```python
from build123d import *

# Parameters (mm, degrees)
CROQUIS1_W              = 60.5
CROQUIS1_H              = 54.5
SALIENTE_EXTRUIR1_DEPTH = 25
CROQUIS2_W              = 56.9
CROQUIS2_H              = 50.9
CORTAR_EXTRUIR1_DEPTH   = 15
CROQUIS3_R              = 2.1
CORTAR_EXTRUIR2_DEPTH   = 5
CORTAR_EXTRUIR3_DEPTH   = 5
CORTAR_EXTRUIR4_DEPTH   = 1.8
CORTAR_EXTRUIR6_START   = -1.8
CORTAR_EXTRUIR6_DEPTH   = 60.5
CROQUIS10_W             = 6
CROQUIS10_H             = 6
CROQUIS10_R             = 1.6
SALIENTE_EXTRUIR2_DEPTH = 3
CROQUIS11_W             = 58.5
CROQUIS11_H             = 52.5
CORTAR_EXTRUIR7_DEPTH   = 15


with BuildPart() as part:
    # Croquis1 → Saliente-Extruir1 (new body)
    with BuildSketch(Plane.XY):
        with Locations((-43.305557703, 3.094674556)):
            Rectangle(CROQUIS1_W, CROQUIS1_H)
    extrude(amount=SALIENTE_EXTRUIR1_DEPTH)

    # Croquis2 → Cortar-Extruir1 (cut)
    with BuildSketch(Plane.XY.offset(25)):
        with Locations((-43.305557703, 3.094674556)):
            Rectangle(CROQUIS2_W, CROQUIS2_H)
    extrude(amount=-CORTAR_EXTRUIR1_DEPTH, mode=Mode.SUBTRACT)

    # Croquis3 → Cortar-Extruir2 (cut)
    with BuildSketch(Plane.XY.offset(10)):
        with Locations((-68.955557703, 25.744674556)):
            Circle(CROQUIS3_R)
        with Locations((-55.855557703, -19.355325444)):
            Circle(CROQUIS3_R)
        with Locations((-30.755557703, -19.355325444)):
            Circle(CROQUIS3_R)
        with Locations((-17.655557703, 25.744674556)):
            Circle(CROQUIS3_R)
        Polygon((-71.755557703, 20.544674556), (-71.755557703, -22.355325444), (-59.855557703, -22.355325444), (-59.855557703, -14.355325444), (-51.855557703, -14.355325444), (-51.855557703, -22.355325444), (-34.755557703, -22.355325444), (-34.755557703, -14.355325444), (-26.755557703, -14.355325444), (-26.755557703, -22.355325444), (-14.855557703, -22.355325444), (-14.855557703, 20.544674556), (-22.855557703, 20.544674556), (-22.855557703, 28.544674556), (-63.755557703, 28.544674556), (-63.755557703, 20.544674556), align=None)
    extrude(amount=-CORTAR_EXTRUIR2_DEPTH, mode=Mode.SUBTRACT)

    # Croquis5 → Cortar-Extruir3 (cut)
    with BuildSketch(Plane(origin=(0, -22.355325444, 0), x_dir=(1, 0, 0), z_dir=(0, 1, 0))):
        with BuildLine():
            Line((-18.605557703, -18), (-18.605557703, -25))
            Line((-18.605557703, -25), (-26.105557703, -25))
            Line((-26.105557703, -25), (-26.105557703, -18))
            ThreePointArc((-26.105557703, -18), (-22.355557703, -14.25), (-18.605557703, -18))
        make_face()
        with BuildLine():
            Line((-39.605557703, -18), (-39.605557703, -25))
            Line((-39.605557703, -25), (-47.105557703, -25))
            Line((-47.105557703, -25), (-47.105557703, -18))
            ThreePointArc((-47.105557703, -18), (-43.355557703, -14.25), (-39.605557703, -18))
        make_face()
        with BuildLine():
            Line((-60.605557703, -18), (-60.605557703, -25))
            Line((-60.605557703, -25), (-68.105557703, -25))
            Line((-68.105557703, -25), (-68.105557703, -18))
            ThreePointArc((-68.105557703, -18), (-64.355557703, -14.25), (-60.605557703, -18))
        make_face()
    extrude(amount=-CORTAR_EXTRUIR3_DEPTH, mode=Mode.SUBTRACT)

    # Croquis6 → Cortar-Extruir4 (cut)
    with BuildSketch(Plane.XZ.offset(-28.544674556)):
        Polygon((-64.805557703, 17), (-21.805557703, 17), (-21.805557703, 10), (-22.855557703, 10), (-22.855557703, 5), (-30.855557703, 5), (-30.855557703, 10), (-64.805557703, 10), align=None)
    extrude(amount=-CORTAR_EXTRUIR4_DEPTH, mode=Mode.SUBTRACT)

    # Croquis9 → Cortar-Extruir6 (cut)
    with BuildSketch(Plane(origin=(-71.755557703, 0, 0), x_dir=(0, 0, -1), z_dir=(1, 0, 0)).offset(CORTAR_EXTRUIR6_START)):
        with BuildLine():
            Line((-10, 20.544674556), (-20, 20.544674556))
            ThreePointArc((-20, 20.544674556), (-22.5, 18.044674556), (-20, 15.544674556))
            Line((-20, 15.544674556), (-10, 15.544674556))
            ThreePointArc((-10, 15.544674556), (-7.5, 18.044674556), (-10, 20.544674556))
        make_face()
        with BuildLine():
            Line((-10, 10.544674556), (-20, 10.544674556))
            ThreePointArc((-20, 10.544674556), (-22.5, 8.044674556), (-20, 5.544674556))
            Line((-20, 5.544674556), (-10, 5.544674556))
            ThreePointArc((-10, 5.544674556), (-7.5, 8.044674556), (-10, 10.544674556))
        make_face()
        with BuildLine():
            Line((-10, 0.544674556), (-20, 0.544674556))
            ThreePointArc((-20, 0.544674556), (-22.5, -1.955325444), (-20, -4.455325444))
            Line((-20, -4.455325444), (-10, -4.455325444))
            ThreePointArc((-10, -4.455325444), (-7.5, -1.955325444), (-10, 0.544674556))
        make_face()
        with BuildLine():
            Line((-10, -9.455325444), (-20, -9.455325444))
            ThreePointArc((-20, -9.455325444), (-22.5, -11.955325444), (-20, -14.455325444))
            Line((-20, -14.455325444), (-10, -14.455325444))
            ThreePointArc((-10, -14.455325444), (-7.5, -11.955325444), (-10, -9.455325444))
        make_face()
    extrude(amount=CORTAR_EXTRUIR6_DEPTH, mode=Mode.SUBTRACT)

    # Croquis10 → Saliente-Extruir2 (add)
    with BuildSketch(Plane.XY.offset(25)):
        with Locations((-76.555557703, 27.344674556)):
            Rectangle(CROQUIS10_W, CROQUIS10_H)
        with Locations((-76.555557703, 27.344674556)):
            Circle(CROQUIS10_R, mode=Mode.SUBTRACT)
        with Locations((-10.055557703, 27.344674556)):
            Rectangle(CROQUIS10_W, CROQUIS10_H)
        with Locations((-10.055557703, 27.344674556)):
            Circle(CROQUIS10_R, mode=Mode.SUBTRACT)
        with Locations((-10.055557703, -21.155325444)):
            Rectangle(CROQUIS10_W, CROQUIS10_H)
        with Locations((-10.055557703, -21.155325444)):
            Circle(CROQUIS10_R, mode=Mode.SUBTRACT)
        with Locations((-76.555557703, -21.155325444)):
            Rectangle(CROQUIS10_W, CROQUIS10_H)
        with Locations((-76.555557703, -21.155325444)):
            Circle(CROQUIS10_R, mode=Mode.SUBTRACT)
    extrude(amount=-SALIENTE_EXTRUIR2_DEPTH)

    # Croquis11 → Cortar-Extruir7 (cut)
    with BuildSketch(Plane.XY.offset(25)):
        with Locations((-43.305557703, 3.094674556)):
            Rectangle(CROQUIS11_W, CROQUIS11_H)
    extrude(amount=-CORTAR_EXTRUIR7_DEPTH, mode=Mode.SUBTRACT)


solid = part.part
```
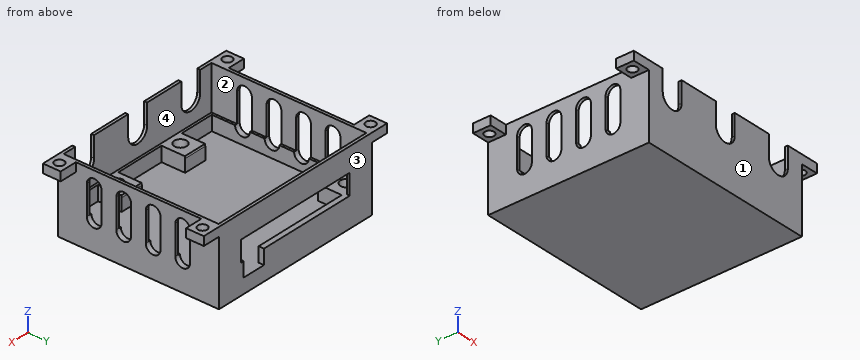
Geometry check sheet. Reference: the model listing, model coordinates, mm. Face numbers are marked on the shaded views. A direction names the side the tool comes from. Coordinates: 2 decimals unless noted, no trailing zeros. Write each loop counter-clockwise with the first axis right and the second up, starting at its lowest first coordinate (ties: lowest second). Pieces come first, ordered by that corner, then holes. Notation, with made-up numbers: (56.5, 29.5) -> (86.5, 29.5) arc R28 cw to (86.5, 56.5) -> close; hole circle Ø3 at (0, -30.75). An arc over 180 degrees is marked (long way). Use CSV: the item, a comma, the result in double quotes. Start each with the question number.
Item 1: Mould release check, pull along X, two halves, no side actions. Record for the marked faces 1 and 2: released by +X, released by -X, zero draft, split by the parting line, or undercut.
Item 2: Cross-section at C-C, the plane z = 12.5. State how many separate pieces and enclosed holes the cut face has, plus the area to 3 significant figures.
Item 3: Set-up check for the marked faces 3 and 4: record each of +Z, -Z, +X, -X, +Y, -Y from which the full face is reachable in a straight line by a thin tool's end or side.
Item 4: Cross-section at A-A, the plane x = -50. Record the cut outline in (y, z).
Item 5: Depth check by flat-ended pin: pin 1 Ø1.1 at (y, z) = (30, 15) entering from -X; pin 2 Ø4 at (x, y) = (-29, 1) entering from +Z; pin 3 Ø0.8 at (y, z) = (-23.5, 20.5) entering from +X. Enter the tip coordinate at first touch or a pass-through.
Item 6: Cross-section at B-B, the plane z = 6. Record the cut outline in (x, y), plus the area to 3 significant figures.
Item 7: Thickness scan on line 1 (X direction, y = -19, z = 11.75); line 2 (X direction, y = -13.5, z = 7.75); line 3 (X direction, y = -18, z = 6.25). Record the ranges inside material, lowest first.
Answers:
1,face 1,"zero draft"
1,face 2,"undercut"
2,separate pieces,"9"
2,enclosed holes,"0"
2,area,"143 mm^2"
3,face 3,"+Z, -Z, +X, -X, +Y"
3,face 4,"+Z"
4,outline,"(-24.16, 0) -> (30.34, 0) -> (30.34, 10) -> (28.54, 10) -> (28.54, 5) -> (-22.36, 5) -> (-22.36, 10) -> (-23.16, 10) -> (-23.16, 25) -> (-24.16, 25) -> close; (29.34, 17) -> (30.34, 17) -> (30.34, 25) -> (29.34, 25) -> close"
5,pin 1,"x = -73.56"
5,pin 2,"z = 5"
5,pin 3,"x = -13.06"
6,outline,"(-73.56, -24.16) -> (-13.06, -24.16) -> (-13.06, 30.34) -> (-22.86, 30.34) -> (-22.86, 20.54) -> (-14.86, 20.54) -> (-14.86, -22.36) -> (-26.76, -22.36) -> (-26.76, -14.36) -> (-34.76, -14.36) -> (-34.76, -22.36) -> (-51.86, -22.36) -> (-51.86, -14.36) -> (-59.86, -14.36) -> (-59.86, -22.36) -> (-71.76, -22.36) -> (-71.76, 20.54) -> (-63.76, 20.54) -> (-63.76, 28.54) -> (-30.86, 28.54) -> (-30.86, 30.34) -> (-73.56, 30.34) -> close; hole circle Ø4.2 at (-68.96, 25.74); hole circle Ø4.2 at (-55.86, -19.36); hole circle Ø4.2 at (-30.76, -19.36); hole circle Ø4.2 at (-17.66, 25.74)"
6,area,"587 mm^2"
7,line 1,"-73.56 to -72.56, -14.06 to -13.06"
7,line 2,"-73.56 to -71.76, -14.86 to -13.06"
7,line 3,"-73.56 to -71.76, -59.86 to -57.46, -54.25 to -51.86, -34.76 to -32.36, -29.15 to -26.76, -14.86 to -13.06"
